Geometry: final body of the model. Coordinates: model frame, mm. A direction names the side the tool comes from. Round coordinates to 2 decimals unless told otherwise and drop trailing zeros. Loops run counter-clockwise (first coordinate to the right, second up) from the corner with the lowest first, then second, coordinate; pieces in that order, holes last. Notation, with made-up numbers: (39, -21.75) - (80, -21.75) arc R30 ccw to (80, 13.25) - close; hole circle Ø6 at (65.25, 41.25). An arc over 180 degrees is marked (long way). Answer in a Markdown table with one row per item. Add a question column.
Autodesk Inventor part; units mm, degrees
ref_plane "YZ Plane" through (0, 0, 0) normal (1, 0, 0) x (0, 1, 0)
ref_plane "XZ Plane" through (0, 0, 0) normal (0, 1, 0) x (-1, 0, 0)
ref_plane "XY Plane" through (0, 0, 0) normal (0, 0, 1) x (1, 0, 0)
sketch "Sketch1" plane through (0, 0, 0) normal (0, 0, 1) x (1, 0, 0)
  circle A0 centre (0, 0) radius 4.7625
  dimension "d0" = 9.525
extrude "Extrusion1" add sketch "Sketch1" along normal blind 84.1375
sketch "Sketch2" plane through (0, 0, 0) normal (0, 0, -1) x (-1, 0, 0)
  point P0 (0, 0)
  point P1 (0, 0)
hole "Hole1" at (0, 0, 0) direction (0, 0, 1) diameter 3.302 depth 12.2936 tip angle 118
chamfer "Chamfer1" distance 0.508 angle 45 1 edges at (-4.7625, 0, 84.1375)
properties part number "post"
1) Section A-A, the plane z = 77. Return the cut outline in (x, y) (1 decimal), and give its area (3 significant figures).
2) Reachability of faces 4 (the cylindrical face through (0.632, 1.525, 6.233)), 5 (the flat face through (0, 0, 84.138)) from +Z, -Z, +X, -X, +Y, -Y: full face, straight path, thin tool, end or side. Return the list, or none.
3) Contact query for flat-ended pins moving along their axis: pin 1 Ø1.5 at (y, z) = (3, 17.5) entering from -X; pin 2 Ø1.5 at (y, z) = (1, 38.5) entering from +X; pin 3 Ø2 at (y, z) = (-2, 69) entering from -X. Output: stop coordinate, or through.
4) Pull-direction query (X, two-part tool) for faces 1 (the conical face through (-0.28, -0.062, 13.113)), 2 (the cylindrical face through (-3.78, 2.9, 41.23)), 3 (the flat face through (2, 0, 0)); classes: pulls with the +X half, pulls with the -X half, needs draft (parallel to the pull), parting line crosses it, or undercut.
5) Material intervals for line 1 along Y through (x, z) = (0, 9.5); line 2 along Z through (x, y) = (-3.25, -2.75); line 3 along X through (y, z) = (0.25, 35), sorted ascending. Write a range as from..to.
Evaluation:
| question | item | result |
|---|---|---|
| 1 | outline | circle Ø9.5 at (0, 0) |
| 1 | area | 71.3 mm² |
| 2 | face 4 | -Z |
| 2 | face 5 | +Z, +X, -X, +Y, -Y |
| 3 | pin 1 | stops at x = -4.2 |
| 3 | pin 2 | stops at x = 4.76 |
| 3 | pin 3 | stops at x = -4.66 |
| 4 | face 1 | undercut |
| 4 | face 2 | parting line crosses it |
| 4 | face 3 | needs draft |
| 5 | line 1 | y = -4.76..-1.65, 1.65..4.76 |
| 5 | line 2 | z = 0..84.13 |
| 5 | line 3 | x = -4.76..4.76 |
